Design review of the part built by this model. Coordinates are the model's own, in mm. A direction names the side the tool comes from. Round coordinates to 2 decimals unless told otherwise and drop trailing zeros. Loops run counter-clockwise (first coordinate to the right, second up) from the corner with the lowest first, then second, coordinate; pieces in that order, holes last. Notation, with made-up numbers: M 67.5,19 L 120.5,19 A29 ccw 120.5,49 Z; hole C 20,-7 d9. An arc over 180 degrees is marked long. Answer as CSV lines item,"result". Start each with the question number.
from build123d import *

# Parameters (mm, degrees)
ESQUISSE1_R                  = 10.5
BOSS_EXTRU_1_DEPTH           = 25
ENL_V_START                  = -15
ENL_V_MAT_EXTRU_1_DEPTH      = 35
ENL_V_MAT_EXTRU_2_DEPTH      = 50
ENL_V_MAT_EXTRU_3_DEPTH      = 15
ESQUISSE1_4_R                = 6.500000002
ENL_V_MAT_EXTRU_4_DEPTH      = 26
ENL_V_MAT_EXTRU_4_DEPTH_BACK = 1
ESQUISSE1_5_R                = 10.000000002
ENL_V_MAT_EXTRU_5_DEPTH      = 12


with BuildPart() as part:
    # Esquisse1 → Boss.-Extru.1 (new body)
    with BuildSketch(Plane.XY):
        with BuildLine():
            Line((600, -25), (0, -25))
            ThreePointArc((0, -25), (-25, 0), (0, 25))
            Line((0, 25), (600, 25))
            ThreePointArc((600, 25), (625, 0), (600, -25))
        make_face()
        Circle(ESQUISSE1_R, mode=Mode.SUBTRACT)
        with BuildLine():
            Line((560, 10.5), (600, 10.5))
            ThreePointArc((600, 10.5), (610.5, 0), (600, -10.5))
            Line((600, -10.5), (560, -10.5))
            ThreePointArc((560, -10.5), (549.5, 0), (560, 10.5))
        make_face(mode=Mode.SUBTRACT)
    extrude(amount=BOSS_EXTRU_1_DEPTH)

    # Esquisse2 → Enl_v. mat.-Extru.1 (cut)
    with BuildSketch(Plane(origin=(0, 25, 0), x_dir=(1, 0, 0), z_dir=(0, 1, 0)).offset(ENL_V_START)):
        Polygon((510, 0), (500, 0), (500, -5), (495, -5), (495, -10), (515, -10), (515, -5), (510, -5), align=None)
    extrude(amount=-ENL_V_MAT_EXTRU_1_DEPTH, mode=Mode.SUBTRACT)

    # Esquisse3 → Enl_v. mat.-Extru.2 (cut)
    with BuildSketch(Plane.XZ.offset(25)):
        Polygon((19.5, 0), (19.5, 5), (14.5, 5), (14.5, 10), (34.5, 10), (34.5, 5), (29.5, 5), (29.5, 0), align=None)
    extrude(amount=-ENL_V_MAT_EXTRU_2_DEPTH, mode=Mode.SUBTRACT)

    # Esquisse1_3 → Enl_v. mat.-Extru.3 (cut)
    with BuildSketch(Plane.XY):
        Polygon((55, 25), (45, 25), (45, 15), (62.5, 15), (62.5, 20), (55, 20), align=None)
        Polygon((310, 20), (310, 25), (290, 25), (290, 20), (282.5, 20), (282.5, 15), (317.5, 15), (317.5, 20), align=None)
        Polygon((555, 15), (555, 25), (545, 25), (545, 20), (537.5, 20), (537.5, 15), align=None)
    extrude(amount=ENL_V_MAT_EXTRU_3_DEPTH, mode=Mode.SUBTRACT)

    # Esquisse1_4 → Enl_v. mat.-Extru.4 (cut, two sides)
    with BuildSketch(Plane.XY) as enl_v_mat_extru_4_sk:
        with Locations((300, 0)):
            Circle(ESQUISSE1_4_R)
        with Locations((450, 0)):
            Circle(ESQUISSE1_4_R)
        with Locations((150, 0)):
            Circle(ESQUISSE1_4_R)
    extrude(amount=ENL_V_MAT_EXTRU_4_DEPTH, mode=Mode.SUBTRACT)
    extrude(enl_v_mat_extru_4_sk.sketch, amount=-ENL_V_MAT_EXTRU_4_DEPTH_BACK, mode=Mode.SUBTRACT)

    # Esquisse1_5 → Enl_v. mat.-Extru.5 (cut)
    with BuildSketch(Plane.XY):
        with Locations((300, 0)):
            Circle(ESQUISSE1_5_R)
        with Locations((450, 0)):
            Circle(ESQUISSE1_5_R)
        with Locations((150, 0)):
            Circle(ESQUISSE1_5_R)
    extrude(amount=ENL_V_MAT_EXTRU_5_DEPTH, mode=Mode.SUBTRACT)


solid = part.part
Item 1: Tool access review of faces 1 (the face through (580, 10.5, 12)), 2 (the face through (450, -7, 12)), 3 (the face through (555, 20, 7)): name each direction out of +Z, -Z, +X, -X, +Y, -Y from which nothing blocks a thin tool from reaching the whole face with its end or side.
Item 2: The part is to be moulded in two halves that separate along Y. For faces 4 (the face through (296, 25, 18)), 5 (the face through (505, -7, 10)), 6 (the face through (549.5, -0.2, 12.3)), 7 (the face through (624.994, 0.55, 12.325)), say which applies: +Y half, -Y half, draft (parallel to the pull), parting line (faces both ways), or undercut.
Item 3: Consider section A-A, the plane x = 450. Write out the cut boundary in (y, z), then the cut area to 3 significant figures.
Item 4: Insertion check: pin 1 Ø5.5 at (y, z) = (22, 9) entering from +X; pin 2 Ø8 at (y, z) = (-15, 13.5) entering from -X; pin 3 Ø5 at (y, z) = (19, 11.5) entering from +X. Each pin has a flat end and moves straight along its axis. Give the tip position at first contact, or say it passes through.
Item 5: Consider section C-C, the plane x = 300. Write out the cut boundary in (y, z), then the cut area to 3 significant figures.
Item 6: Consider section B-B, the plane y = 0. Count the separate pieces of the cut face and the enclosed holes in it, then the cut area to 3 significant figures.
Item 7: To check wall thickness, follow line 1 (X direction, y = -0.5, z = 12.5) (3 decimals); line 2 (Y direction, x = 150, z = 6); line 3 (Y direction, x = 450, z = 20). State the ranges of each line that lie inside material, in increasing order.
Found:
1,face 1,"+Z, -Z"
1,face 2,"-Z"
1,face 3,"-Z, +Y"
2,face 4,"+Y half"
2,face 5,"draft"
2,face 6,"undercut"
2,face 7,"parting line"
3,outline,"M -25,0 L -10,0 L -10,12 L -6.5,12 L -6.5,25 L -25,25 Z; M 6.5,12 L 10,12 L 10,0 L 25,0 L 25,25 L 6.5,25 Z"
3,area,"841 mm^2"
4,pin 1,"stops at x = 615.95"
4,pin 2,"stops at x = -22.45"
4,pin 3,"stops at x = 618.78"
5,outline,"M -25,0 L -10,0 L -10,12 L -6.5,12 L -6.5,25 L -25,25 Z; M 6.5,12 L 10,12 L 10,0 L 15,0 L 15,15 L 25,15 L 25,25 L 6.5,25 Z"
5,area,"691 mm^2"
6,separate pieces,"6"
6,enclosed holes,"0"
6,area,"12,700 mm^2"
7,line 1,"x = -24.995 to -10.488, 10.488 to 143.519, 156.481 to 293.519, 306.481 to 443.519, 456.481 to 549.512, 610.488 to 624.995"
7,line 2,"y = -25 to -10, 10 to 25"
7,line 3,"y = -25 to -6.5, 6.5 to 25"
